For this review, take the finished solid that the model builds, in its own axes (mm). A direction names the side the tool comes from. Coordinates: 2 decimals unless noted, no trailing zeros. Loops run counter-clockwise (first coordinate to the right, second up) from the corner with the lowest first, then second, coordinate; pieces in that order, holes last. Notation, with made-up numbers: M -36.5,24 L 5.5,24 A8 cw 5.5,33 Z; hole C 14.25,12 d5. An arc over 180 degrees is marked long. Answer as a JSON object with one key per item and string values. Group by question number.
Item 1: Wall thickness on L1, parallel to Y at x = 84.5, z = 50; L2, parallel to X at y = 65, z = 89.5; L3, parallel to Y at x = 68.5, z = 68.5: over which ranges is each line inside the solid? List them lowest first. Write a range as from..to.
Item 2: Mouldability with a two-part tool opening along X and no side actions: class faces 1 (the face through (100, 72, 17)), 2 (the face through (60.5, 11.286, 50.7)), 3 (the face through (72, 16, 0)), 4 (the face through (0, 72, 17)) as +X half, -X half, draft (parallel to the pull), parting line (faces both ways), or undercut.
Item 3: Add section B-B (z = 50). State the section outline as (x, y) points, then the cut area to 3 significant figures.
Item 4: Insertion check: pin 1 (4 mm diameter, centred on y = 52, z = 86.5, fed in from -X); pin 2 (12 mm diameter, centred on y = 25, z = 33, fed in from -X) (3 decimals). Each pin has a flat end and moves straight along its axis. Give the tip position at first contact, or say it passes through.
Item 5: Tool access review of faces 5 (the face through (88.777, 50, 8)), 6 (the face through (72, 16, 100)): name each direction out of +Z, -Z, +X, -X, +Y, -Y from which nothing blocks a thin tool from reaching the whole face with its end or side.
Item 6: Add section A-A (y = 50). State the section outline as (x, z) points, then the cut area to 3 significant figures.
Item 7: Add section D-D (z = 92.5). State the section outline as (x, y) points.
Item 8: Add section C-C (x = 60.5). State the section outline as (y, z) points.
from build123d import *

# Parameters (mm, degrees)
F0_W     = 100
F0_H     = 100
F1_DEPTH = 100
F2_R     = 36.715215
F3_DEPTH = 100
F5_DEPTH = 100.001


with BuildPart() as f1:
    # F0 (on Right) → F1 (new body)
    with BuildSketch(Plane.YZ):
        with Locations((50, 50)):
            Rectangle(F0_W, F0_H)
    extrude(amount=F1_DEPTH)

    # F2 (on face) → F3 (cut, through all)
    with BuildSketch(Plane.YZ.offset(100)):
        with Locations((50, 50)):
            Circle(F2_R)
    extrude(amount=-F3_DEPTH, mode=Mode.SUBTRACT)

    # F4 (on face) → F5 (cut, through all)
    with BuildSketch(Plane.XY.offset(100)):
        Polygon((88.777177, 27.611986), (88.777177, 72.388014), (50, 94.776027), (11.222823, 72.388014), (11.222823, 27.611986), (50, 5.223973), align=None)
    extrude(amount=-F5_DEPTH, mode=Mode.SUBTRACT)


solid = f1.part
From the geometry:
{
 "1": {"L1": "y = 0..13.28, 86.72..100", "L2": "x = 0..11.22, 88.78..100", "L3": "y = 0..15.9, 84.1..100"},
 "2": {"face 1": "+X half", "face 2": "undercut", "face 3": "draft", "face 4": "-X half"},
 "3": {"outline": "M 0,0 L 100,0 L 100,13.28 L 63.96,13.28 L 50,5.22 L 36.04,13.28 L 0,13.28 Z; M 0,86.72 L 36.04,86.72 L 50,94.78 L 63.96,86.72 L 100,86.72 L 100,100 L 0,100 Z", "area": "2,430 mm²"},
 "4": {"pin 1": "stops at x = 0", "pin 2": "passes through"},
 "5": {"face 5": "+Z, -Z", "face 6": "+Z, +X, -X, +Y, -Y"},
 "6": {"outline": "M 0,0 L 11.22,0 L 11.22,13.28 L 0,13.28 Z; M 0,86.72 L 11.22,86.72 L 11.22,100 L 0,100 Z; M 88.78,0 L 100,0 L 100,13.28 L 88.78,13.28 Z; M 88.78,86.72 L 100,86.72 L 100,100 L 88.78,100 Z", "area": "596 mm²"},
 "7": {"outline": "M 0,0 L 100,0 L 100,100 L 0,100 Z; hole M 11.22,27.61 L 50,5.22 L 88.78,27.61 L 88.78,72.39 L 50,94.78 L 11.22,72.39 Z"},
 "8": {"outline": "M 0,0 L 11.29,0 L 11.29,100 L 0,100 Z; M 88.71,0 L 100,0 L 100,100 L 88.71,100 Z"}
}
